Could you check a few things on this model? Use its own coordinates, in mm. Give positions to 0.01 mm unless a question says otherwise; leave off trailing zeros. Order: outer loops, then holes, each group sorted by start corner. A loop starts at its lowest first (then second) coordinate and runs counter-clockwise, first axis right, second up.
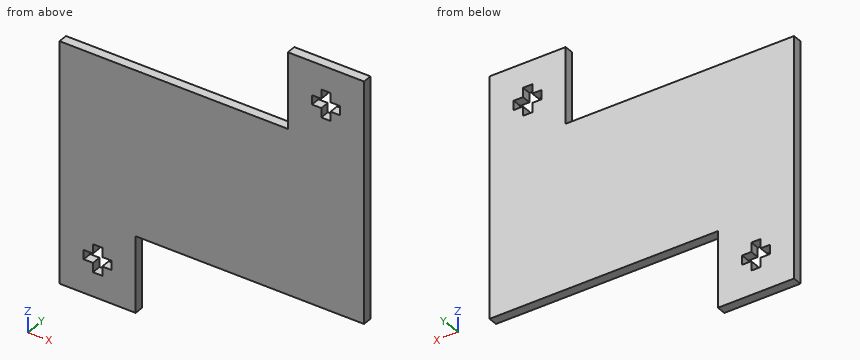
from build123d import *

# Parameters (mm, degrees)
BOSS_EXTRUDE1_DEPTH = 5.08


with BuildPart() as part:
    # Sketch1 → Boss-Extrude1 (new body)
    with BuildSketch(Plane(origin=(0, 0, 0), x_dir=(1, 0, 0), z_dir=(0, 1, 0))):
        Polygon((-36.363267323, 33.553843074), (88.708872677, 33.553843074), (88.708872677, -56.605996926), (88.708872677, -98.295016926), (47.014772677, -98.295016926), (47.014772677, -56.605996926), (-78.052287323, -56.605996926), (-78.052287323, 33.553843074), (-78.052287323, 75.242863074), (-36.363267323, 75.242863074), align=None)
        Polygon((-57.207777323, 62.018353074), (-54.667777323, 62.018353074), (-54.667777323, 56.938353074), (-49.587777323, 56.938353074), (-49.587777323, 54.398353074), (-49.587777323, 51.858353074), (-54.667777323, 51.858353074), (-54.667777323, 46.778353074), (-57.207777323, 46.778353074), (-59.747777323, 46.778353074), (-59.747777323, 51.858353074), (-64.827777323, 51.858353074), (-64.827777323, 54.398353074), (-64.827777323, 56.938353074), (-59.747777323, 56.938353074), (-59.747777323, 62.018353074), align=None, mode=Mode.SUBTRACT)
        Polygon((60.241822677, -77.450506926), (60.241822677, -74.910506926), (65.321822677, -74.910506926), (65.321822677, -69.830506926), (67.861822677, -69.830506926), (70.401822677, -69.830506926), (70.401822677, -74.910506926), (75.481822677, -74.910506926), (75.481822677, -77.450506926), (75.481822677, -79.990506926), (70.401822677, -79.990506926), (70.401822677, -85.070506926), (67.861822677, -85.070506926), (65.321822677, -85.070506926), (65.321822677, -79.990506926), (60.241822677, -79.990506926), align=None, mode=Mode.SUBTRACT)
    extrude(amount=BOSS_EXTRUDE1_DEPTH)


solid = part.part
Item 1: Please list where these lines run through material, in increasing order: line 1 along X through (y, z) = (2.4, -49); line 2 along Z through (x, y) = (60.5, 3.35); line 3 along Z through (x, y) = (-59.5, 3.95).
Findings:
line 1: x = -78.05 to -59.75, -54.67 to -36.36
line 2: z = -33.55 to 74.91, 79.99 to 98.3
line 3: z = -75.24 to -62.02, -46.78 to 56.61
Item 2: Imagine slicing it at B-B on x = 11.5. List the corners of the cut face in (y, z) for me, then the cut area to 3 significant figures.
Findings:
outline: (0, -33.55) - (5.08, -33.55) - (5.08, 56.61) - (0, 56.61) - close
area: 458 mm2
Item 3: Imagine slicing it at A-A on y = 3.8. Give the number of separate pieces and of enclosed holes in the cut face, then the cut area to 3 significant figures.
Findings:
separate pieces: 1
enclosed holes: 2
area: 18,300 mm2
Item 4: Imagine slicing it at C-C on z = 88.5. List the corners of the cut face in (x, y) for me.
Findings:
outline: (47.01, 0) - (88.71, 0) - (88.71, 5.08) - (47.01, 5.08) - close
Item 5: For pin 1 (2.5 mm diameter, centred on x = -62.5, y = 3, fed in from +Z); pin 2 (1 mm diameter, centred on x = 46.5, z = -28, fed in from -Y); pin 3 (3 mm diameter, centred on x = -23, y = 2, fed in from -Z); pin 4 (1.5 mm diameter, centred on y = 2, z = 72.5, fed in from -X), each with a flat end and sliding along its axis, tell me the tip position at first contact or that it passes through.
Findings:
pin 1: stops at z = 56.61
pin 2: stops at y = 0
pin 3: stops at z = -33.55
pin 4: stops at x = 47.01
